Autodesk Inventor part; units mm, degrees
ref_plane "YZ Plane" through (0, 0, 0) normal (1, 0, 0) x (0, 1, 0)
ref_plane "XZ Plane" through (0, 0, 0) normal (0, 1, 0) x (-1, 0, 0)
ref_plane "XY Plane" through (0, 0, 0) normal (0, 0, 1) x (1, 0, 0)
sketch "Sketch1" plane through (0, 0, 0) normal (0, 0, 1) x (1, 0, 0)
  circle A0 centre (0, 0) radius 9.5
  dimension "d0" = 19
extrude "Extrusion1" add sketch "Sketch1" against normal blind 24.5
sketch "Sketch2" plane through (0, 0, -24.5) normal (0, 0, -1) x (-1, 0, 0)
  circle A0 centre (0, 0) radius 8
  dimension "d3" = 16
extrude "Extrusion2" add sketch "Sketch2" along normal blind 15
sketch "Sketch3" plane through (0, 0, 0) normal (0, 0, 1) x (1, 0, 0)
  line L0 (0, 0) -> (0, 8.75)
  line L1 (0, 8.75) -> (1.75, 8.75)
  line L2 (1.75, 8.75) -> (1.75, 1.75)
  line L3 (1.75, 1.75) -> (8.75, 1.75)
  line L4 (8.75, 1.75) -> (8.75, -1.75)
  line L5 (8.75, -1.75) -> (1.75, -1.75)
  line L6 (1.75, -1.75) -> (1.75, -8.75)
  line L7 (1.75, -8.75) -> (-1.75, -8.75)
  line L8 (-1.75, -8.75) -> (-1.75, -1.75)
  line L9 (-1.75, -1.75) -> (-8.75, -1.75)
  line L10 (-8.75, -1.75) -> (-8.75, 1.75)
  line L11 (-8.75, 1.75) -> (-1.75, 1.75)
  line L12 (-1.75, 1.75) -> (-1.75, 8.75)
  line L13 (-1.75, 8.75) -> (0, 8.75)
  dimension "d26" = 8.75
  dimension "d27" = 1.75
  dimension "d28" = 7
  dimension "d29" = 7
  dimension "d30" = 3.5
  dimension "d31" = 7
  dimension "d33" = 7
  dimension "d34" = 3.5
  dimension "d35" = 7
  dimension "d36" = 7
  dimension "d37" = 3.5
  dimension "d38" = 7
  dimension "d39" = 7
extrude "Extrusion3" add sketch "Sketch3" along normal blind 5
sketch "Sketch4" plane through (0, 0, 5) normal (0, 0, 1) x (1, 0, 0)
  circle A0 centre (0, 0) radius 1.3
  dimension "d23" = 2.6
extrude "Extrusion4" cut sketch "Sketch4" against normal blind 42.9375
properties part number "OmniWheelAxleRear"
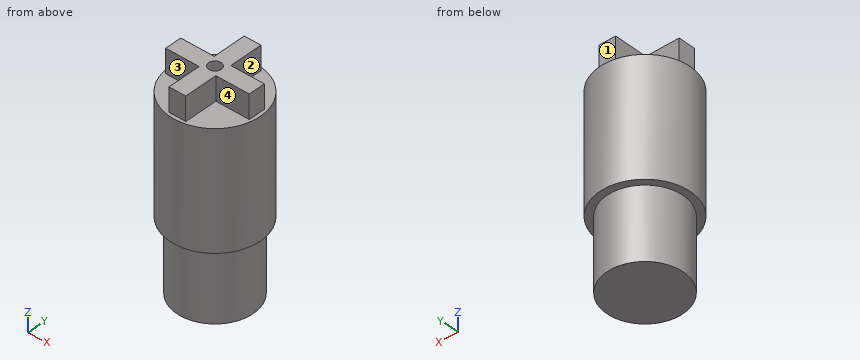
Design review of the part built by this model. Coordinates are the model's own, in mm. Face numbers are marked on the shaded views. A direction names the side the tool comes from. Coordinates: 2 decimals unless noted, no trailing zeros. Write each loop counter-clockwise with the first axis right and the second up, starting at its lowest first coordinate (ties: lowest second). Pieces come first, ordered by that corner, then holes. Notation, with made-up numbers: M 50.25,-14 L 81.25,-14 A11 ccw 81.25,4 Z; hole C 14,-7.5 d11. An arc over 180 degrees is marked long. Answer as a JSON object with one key per item and string values.
Item 1: Insertion check: pin 1 Ø1.5 at (x, z) = (4, 3.5) entering from -Y; pin 2 Ø3 at (x, z) = (2, -29) entering from +Y; pin 3 Ø4 at (x, z) = (3.5, -33) entering from -Y. Each pin has a flat end and moves straight along its axis. Give the tip position at first contact, or say it passes through.
Outcome:
{"pin 1": "y = -1.75", "pin 2": "y = 7.98", "pin 3": "y = -7.86"}
Item 2: Wall thickness on probe 1 along Y at (x, z) = (0, -4); probe 2 along Y at (x, z) = (0, -28); probe 3 along X at (y, z) = (-1, -3): over which ranges is each line inside the solid? List them lowest first.
Outcome:
{"probe 1": "-9.5 to -1.3, 1.3 to 9.5", "probe 2": "-8 to -1.3, 1.3 to 8", "probe 3": "-9.45 to -0.83, 0.83 to 9.45"}
Item 3: Add section A-A, the plane x = 0. Give the boundary of the cut face in (y, z), and give its area (3 significant figures).
Outcome:
{"outline": "M -9.5,-24.5 L -8,-24.5 L -8,-39.5 L 8,-39.5 L 8,-24.5 L 9.5,-24.5 L 9.5,0 L 8.75,0 L 8.75,5 L 1.3,5 L 1.3,-37.94 L -1.3,-37.94 L -1.3,5 L -8.75,5 L -8.75,0 L -9.5,0 Z", "area": "681 mm²"}
Item 4: Add section C-C, the plane z = -31.5. Give the boundary of the cut face in (x, y).
Outcome:
{"outline": "C 0,0 d16; hole C 0,0 d2.6"}
Item 5: Machinability: for the marked faces 1, 2, 3 and 4, which of the approach directions +Z, -Z, +X, -X, +Y, -Y give a long, thin tool a straight path to every point of the face, cutting with its end or side? Answer none if there is none.
Outcome:
{"face 1": "+Z, +X, -X, +Y", "face 2": "+Z, +X, +Y", "face 3": "+Z, -X, -Y", "face 4": "+Z, +X, -Y"}
Item 6: Add section D-D, the plane y = -6. Give the boundary of the cut face in (x, z), and give its area (3 significant figures).
Outcome:
{"outline": "M -7.37,-24.5 L -5.29,-24.5 L -5.29,-39.5 L 5.29,-39.5 L 5.29,-24.5 L 7.37,-24.5 L 7.37,0 L 1.75,0 L 1.75,5 L -1.75,5 L -1.75,0 L -7.37,0 Z", "area": "537 mm²"}
